The model under review builds one solid part; all positions refer to its coordinate system, in mm. A direction names the side the tool comes from. Round coordinates to 2 decimals unless told otherwise and drop trailing zeros. Write each loop counter-clockwise with the first axis right and the second up, starting at its lowest first coordinate (ties: lowest second). Pieces come first, ordered by that corner, then holes. Notation, with made-up numbers: (66.5, 4) - (93.5, 4) arc R13 cw to (93.5, 20) - close; hole circle Ø6 at (-12.75, 53). An arc over 180 degrees is marked (long way). Return JSON: item names as keys, results as strings.
Autodesk Inventor part; units mm, degrees
ref_plane "YZ Plane" through (0, 0, 0) normal (1, 0, 0) x (0, 1, 0)
ref_plane "XZ Plane" through (0, 0, 0) normal (0, 1, 0) x (-1, 0, 0)
ref_plane "XY Plane" through (0, 0, 0) normal (0, 0, 1) x (1, 0, 0)
sketch "Sketch1" plane through (0, 0, 0) normal (0, 0, 1) x (1, 0, 0)
  circle A0 centre (0, 0) radius 3
  dimension "d0" = 6
extrude "Extrusion1" add sketch "Sketch1" along normal mid plane 74
sketch "Sketch2" plane through (0, 0, 37) normal (0, 0, 1) x (1, 0, 0)
  circle A0 centre (0, 0) radius 3
  circle A1 centre (0, 0) radius 2
  dimension "d3" = 4
extrude "Extrusion2" add sketch "Sketch2" along normal blind 15 contours A1
ref_plane "Work Plane1" through (0, 0, 0) normal (0, 0, 1) x (1, 0, 0)
mirror "Mirror1" about plane through (0, 0, 0) normal (0, 0, 1) of "Extrusion2"
ref_plane "Work Plane2" through (0, 0, 0) normal (0, 0, 1) x (1, 0, 0)
properties part number "four"
(1) Add section D-D (z = 22.5). Write out the cut boundary in (x, y), plus the area to 3 significant figures.
Filled in:
{"outline": "circle Ø6 at (0, 0)", "area": "28.3 mm2"}
(2) Add section B-B (x = 0). Write out the cut boundary in (y, z).
Filled in:
{"outline": "(-3, -37) - (-2, -37) - (-2, -52) - (2, -52) - (2, -37) - (3, -37) - (3, 37) - (2, 37) - (2, 52) - (-2, 52) - (-2, 37) - (-3, 37) - close"}
(3) Clearance check with a flat-ended pin moving along its axis: pin 1 Ø1.5 at (x, y) = (-2, 2) entering from +Z. State where the tip first meets the part, or that it passes through.
Filled in:
{"pin 1": "stops at z = 37"}
(4) Add section C-C (z = 40). Write out the cut boundary in (x, y), plus the area to 3 significant figures.
Filled in:
{"outline": "circle Ø4 at (0, 0)", "area": "12.6 mm2"}
(5) Wall thickness on line 1 (Z direction, x = 0.55, y = -2.6); line 2 (Y direction, x = -0.1, z = -23); line 3 (Y direction, x = 1.6, z = 9): over which ranges is each line inside the solid? List them lowest first.
Filled in:
{"line 1": "z = -37 to 37", "line 2": "y = -3 to 3", "line 3": "y = -2.54 to 2.54"}
(6) For faces 1 (the flat face through (1, -2, -37)), 2 (the cylindrical face through (0, 2, 44)), 3 (the flat face through (0, 0, -52)), list the 3-axis set-ups (+Z, -Z, +X, -X, +Y, -Y) from which the entire face can be reached by the end or side of a thin tool; tool diameter is ignored.
Filled in:
{"face 1": "-Z", "face 2": "+Z", "face 3": "-Z, +X, -X, +Y, -Y"}
(7) Mouldability with a two-part tool opening along X and no side actions: class faces 4 (the cylindrical face through (-3, 0, 1)), 5 (the flat face through (0, 0, 52)) as released by +X, released by -X, zero draft, split by the parting line, or undercut.
Filled in:
{"face 4": "split by the parting line", "face 5": "zero draft"}
(8) Add section A-A (y = -0.95). Write out the cut boundary in (x, z).
Filled in:
{"outline": "(-2.85, -37) - (-1.76, -37) - (-1.76, -52) - (1.76, -52) - (1.76, -37) - (2.85, -37) - (2.85, 37) - (1.76, 37) - (1.76, 52) - (-1.76, 52) - (-1.76, 37) - (-2.85, 37) - close"}
